Autodesk Inventor part; units mm, degrees
ref_plane "YZ Plane" through (0, 0, 0) normal (1, 0, 0) x (0, 1, 0)
ref_plane "XZ Plane" through (0, 0, 0) normal (0, 1, 0) x (-1, 0, 0)
ref_plane "XY Plane" through (0, 0, 0) normal (0, 0, 1) x (1, 0, 0)
sketch "Эскиз5" plane through (0, 0, 0) normal (0, 1, 0) x (-1, 0, 0)
  line L0 (152.615, 60) -> (152.615, -3)
  line L1 (152.615, -3) -> (0, -3)
  line L2 (0, -3) -> (0, 0)
  line L3 (0, 0) -> (149.615, 0)
  line L4 (149.615, 0) -> (149.615, 60)
  line L5 (149.615, 60) -> (152.615, 60)
  dimension "d40" = 149.615
  dimension "d41" = 3
  dimension "d42" = 60
extrude "Выдавливание2" add sketch "Эскиз5" along normal blind 10
sketch "Эскиз6" plane through (-149.615, 0, 60) normal (1, 0, 0) x (0, 0, -1)
  line L0 (63, 0) -> (0, 0)
  line L1 (0, 10) -> (10, 10) construction
  line L2 (10, 10) -> (10, 0) construction
  line L3 (10, 0) -> (0, 0) construction
  line L4 (0, 0) -> (0, 10) construction
  line L5 (0, 10) -> (10, 0) construction
  line L6 (10, 10) -> (0, 0) construction
  circle A0 centre (5, 5) radius 23
  point P0 (60, 0)
  dimension "d45" = 46
extrude "Выдавливание3" add sketch "Эскиз6" against normal blind 3
properties part number "Mirror_ыефтв" material "Сталь, мягкая"
Here's how the part is built. I have some questions about the finished solid (model axes, mm). A direction names the side the tool comes from. Give positions to 0.01 mm unless a question says otherwise; leave off trailing zeros. Loops run counter-clockwise (first coordinate to the right, second up) from the corner with the lowest first, then second, coordinate; pieces in that order, holes last. Notation, with made-up numbers: (34.5, 27) -> (67.5, 27) arc R31 ccw to (67.5, 56) -> close; hole circle Ø10 at (-13.5, 73.5). An arc over 180 degrees is marked (long way). Answer as a JSON object with one key per item and string values. Group by question number.
Item 1: Will these pins go through, and if not, where does the flat tip stop? pin 1 (10.5 mm diameter, centred on x = -97, z = 7, fed in from +Y); pin 2 (8 mm diameter, centred on y = -12, z = 43, fed in from +X) (3 decimals); pin 3 (3 mm diameter, centred on x = -92, y = -1, fed in from +Z).
Item 2: I need wall thicknesses on L1, parallel to X at y = -4, z = 41 (3 decimals); L2, parallel to Z at x = -62, y = 5.5. Which ranges of each line are inside material? Lowest first, please.
Item 3: Imagine slicing it at A-A on x = -127.5. Write out the boundary of the cut face in (y, z).
Item 4: On a 3-axis mill with a long thin cutter (end or side, diameter ignored), from which of +Z, -Z, +X, -X, +Y, -Y can I reach the whole of each face in a straight line? I mean faces 1 (the flat face through (-149.615, 5, 48)), 2 (the flat face through (-77, 5, -3)). Say none if no direction works.
Item 5: Imagine slicing it at B-B on y = 5. Write out the boundary of the cut face in (x, z) (3 decimals), then the cut area to 3 significant figures.
Item 6: Imagine slicing it at C-C on z = 55. Write out the boundary of the cut face in (x, y) (3 decimals), then the cut area to 3 significant figures.
Answer list:
{
 "1": {"pin 1": "passes through", "pin 2": "stops at x = -149.615", "pin 3": "stops at z = 0"},
 "2": {"L1": "x = -152.615 to -149.615", "L2": "z = -3 to 0"},
 "3": {"outline": "(0, -3) -> (10, -3) -> (10, 0) -> (0, 0) -> close"},
 "4": {"face 1": "+Z, +X, +Y, -Y", "face 2": "-Z, +X, -X, +Y, -Y"},
 "5": {"outline": "(-152.615, -3) -> (0, -3) -> (0, 0) -> (-149.615, 0) -> (-149.615, 78) -> (-152.615, 78) -> close", "area": "692 mm2"},
 "6": {"outline": "(-152.615, -18) -> (-149.615, -18) -> (-149.615, 28) -> (-152.615, 28) -> close", "area": "138 mm2"}
}
